Part model, mm, in its own coordinate system. A direction names the side the tool comes from. Coordinates: 2 decimals unless noted, no trailing zeros. Order: outer loops, then holes, each group sorted by start corner. A loop starts at its lowest first (then second) coordinate and runs counter-clockwise, first axis right, second up.
from build123d import *

# Parameters (mm, degrees)
SKETCH_1_W          = 30
SKETCH_1_H          = 12
EXTRUDE_1_DEPTH     = 6
SKETCH_3_W          = 6
SKETCH_3_H          = 6
CUT_EXTRUDE_1_DEPTH = 3
CUT_EXTRUDE_2_REACH = 20.493
SKETCH_4_R          = 1.65


with BuildPart() as part:
    # 草图1 → 凸台-拉伸1 (new body)
    with BuildSketch(Plane(origin=(0, 0, 0), x_dir=(1, 0, 0), z_dir=(0, 1, 0))):
        with Locations((0, 6)):
            Rectangle(SKETCH_1_W, SKETCH_1_H)
    extrude(amount=EXTRUDE_1_DEPTH)

    # 草图2 → 切除-旋转1 (revolve, cut)
    with BuildSketch(Plane.XY):
        Polygon((-8, 0), (0, 0), (0, 3), (-9, 3), (-9, 1), (-8, 1), align=None)
        Polygon((-9, 3), (0, 3), (0, 6), (-8, 6), (-8, 5), (-9, 5), align=None)
    revolve(axis=Axis((0, 0, 0), (0, 1, 0)), mode=Mode.SUBTRACT)

    # 草图3 → 切除-拉伸1 (cut)
    with BuildSketch(Plane(origin=(0, 0, -12), x_dir=(-1, 0, 0), z_dir=(0, 0, -1))):
        with Locations((-12, 3)):
            Rectangle(SKETCH_3_W, SKETCH_3_H)
    cut_extrude_1 = extrude(amount=-CUT_EXTRUDE_1_DEPTH, mode=Mode.SUBTRACT)

    # 草图4 → 切除-拉伸2 (cut, up to next)
    with BuildSketch(Plane(origin=(0, 0, -9), x_dir=(-1, 0, 0), z_dir=(0, 0, -1)), mode=Mode.PRIVATE) as cut_extrude_2_sk1:
        with Locations((-12, 3)):
            Circle(SKETCH_4_R)
    cut_extrude_2_tool1 = extrude(cut_extrude_2_sk1.sketch, amount=-CUT_EXTRUDE_2_REACH, mode=Mode.PRIVATE) & part.part
    cut_extrude_2 = cut_extrude_2_tool1.solids().sort_by_distance((12, 3, -9))[0]
    add(cut_extrude_2, mode=Mode.SUBTRACT)

    # 镜向1: 切除-拉伸1, 切除-拉伸2 across plane
    add(cut_extrude_1.mirror(Plane(origin=(0, 0, 0), x_dir=(0, 0, 1), z_dir=(1, 0, 0))), mode=Mode.SUBTRACT)
    add(cut_extrude_2.mirror(Plane(origin=(0, 0, 0), x_dir=(0, 0, 1), z_dir=(1, 0, 0))), mode=Mode.SUBTRACT)


solid = part.part
Q1. Wall check: line 1 along Y through (x, z) = (-12, -4); line 2 along Y through (x, z) = (-7.75, -2.25); line 3 along X through (y, z) = (2.65, -1.75). Give the ranges that are in metal, low to high.
Results list:
line 1: y = 0 to 1.35, 4.65 to 6
line 2: y = 0 to 1, 5 to 6
line 3: x = -15 to -13.61, -10.39 to -8.83, 8.83 to 10.39, 13.61 to 15
Q2. Cut at B-B on x = -12. Write the cut outline in (y, z).
Results list:
outline: (0, -9) - (1.35, -9) - (1.35, 0) - (0, 0) - close; (4.65, -9) - (6, -9) - (6, 0) - (4.65, 0) - close
Q3. Cut at A-A on y = 3. Write the cut outline in (x, z), and give its area (3 significant figures).
Results list:
outline: (-15, -9) - (-13.65, -9) - (-13.65, 0) - (-15, 0) - close; (-10.35, -9) - (-9, -9) - (-9, -12) - (9, -12) - (9, -9) - (10.35, -9) - (10.35, 0) - (9, 0) arc R9 cw to (-9, 0) - (-10.35, 0) - close; (13.65, -9) - (15, -9) - (15, 0) - (13.65, 0) - close
area: 137 mm2
Q4. Which spindle directions (+Z, -Z, +X, -X, +Y, -Y) get a long thin tool onto all of the face, cutting with end or side? Do faces 1 (the face through (0, 3, -9)), 2 (the face through (-9, 3, -11)), 3 (the face through (10.7, 4.4, -9)). Say none if no direction does.
Results list:
face 1: +Z
face 2: -Z, -X, +Y, -Y
face 3: -Z, +X, +Y, -Y
Q5. Pin check, flat tips, straight feed: pin 1 Ø3 at (x, y) = (12, 3) entering from +Z; pin 2 Ø1.5 at (y, z) = (3.5, -10) entering from -X; pin 3 Ø1.8 at (x, y) = (-11, 2) entering from -Z. Stop position of each tip, or through.
Results list:
pin 1: passes through
pin 2: stops at x = -9
pin 3: stops at z = -9
Q6. Cut at D-D on y = 5.3. Write the cut outline in (x, z), and give its area (3 significant figures).
Results list:
outline: (-15, -9) - (-9, -9) - (-9, -12) - (9, -12) - (9, -9) - (15, -9) - (15, 0) - (8, 0) arc R8 cw to (-8, 0) - (-15, 0) - close
area: 223 mm2
Q7. Mould opens along Y. For faces 4 (the face through (0, 6, -9)), 5 (the face through (0.04, 1, -8.15)), 6 (the face through (0, 0, -9)) say: pulls with the +Y half, pulls with the -Y half, needs draft (parallel to the pull), parting line crosses it, or undercut.
Results list:
face 4: pulls with the +Y half
face 5: undercut
face 6: pulls with the -Y half
Q8. Cut at C-C on z = -1. Write the cut outline in (x, y), and give its area (3 significant figures).
Results list:
outline: (-15, 0) - (-7.94, 0) - (-7.94, 1) - (-8.94, 1) - (-8.94, 5) - (-7.94, 5) - (-7.94, 6) - (-15, 6) - close; (7.94, 0) - (15, 0) - (15, 6) - (7.94, 6) - (7.94, 5) - (8.94, 5) - (8.94, 1) - (7.94, 1) - close; hole circle Ø3.3 at (-12, 3); hole circle Ø3.3 at (12, 3)
area: 59.6 mm2
